Autodesk Inventor part; units mm, degrees
ref_plane "YZ Plane" through (0, 0, 0) normal (1, 0, 0) x (0, 1, 0)
ref_plane "XZ Plane" through (0, 0, 0) normal (0, 1, 0) x (-1, 0, 0)
ref_plane "XY Plane" through (0, 0, 0) normal (0, 0, 1) x (1, 0, 0)
sketch "Sketch1" plane through (0, 0, 0) normal (0, 0, 1) x (1, 0, 0)
  line L0 (-20, -5) -> (20, -5)
  line L1 (20, -5) -> (20, 5)
  line L2 (20, 5) -> (-20, 5)
  line L3 (-20, 5) -> (-20, -5)
  line L4 (-20, -5) -> (20, 5) construction
  line L5 (20, -5) -> (-20, 5) construction
  circle A0 centre (0, -18) radius 11.15
  circle A1 centre (0, -18) radius 5.25
  circle A2 centre (0, -18) radius 17.5
  line L6 (-20, -5) -> (-17.2455, -20.9738)
  line L7 (20, -5) -> (17.2455, -20.9738)
  circle A3 centre (0, -10) radius 1.65
  circle A4 centre (-8, -18) radius 1.65
  circle A5 centre (0, -26) radius 1.65
  circle A6 centre (8, -18) radius 1.65
  point P0 (0, 0)
  dimension "d0" = 22.3
  dimension "d1" = 10.5
  dimension "d2" = 35
  dimension "d3" = 3.3
  dimension "d4" = 8
  dimension "d7" = 360
  dimension "d14" = 40
  dimension "d16" = 23
  dimension "d17" = 10
extrude "Extrusion1" add sketch "Sketch1" along normal blind 10 contours L3 L2 L1 L0 A2 | L0 A2 L6 | A2 L0 | L0 A2 | L0 L7 A2 | A0
extrude "Extrusion2" cut sketch "Sketch1" along normal blind 3 contours A0
sketch "Sketch2" plane through (0, 0, 10) normal (0, 0, 1) x (1, 0, 0)
  line L0 (20, 5) -> (-20, 5)
  line L1 (-20, 5) -> (-20, -5)
  line L2 (-20, -5) -> (-17.2455, -20.9738)
  arc A0 (-17.2455, -20.9738) -> (17.2455, -20.9738) centre (0, -18) ccw
  line L3 (17.2455, -20.9738) -> (20, -5)
  line L4 (20, -5) -> (20, 5)
  circle A1 centre (0, -18) radius 5.25
  circle A2 centre (0, -10) radius 1.65
  circle A3 centre (-8, -18) radius 1.65
  circle A4 centre (0, -26) radius 1.65
  circle A5 centre (8, -18) radius 1.65
  circle A6 centre (-10, -3) radius 1.65
  circle A7 centre (10, -3) radius 1.65
  line L5 (-10, -3) -> (10, -3)
  point P0 (0, 0)
  point P1 (0, -3)
  dimension "d18" = 3.3
  dimension "d19" = 3.3
  dimension "d20" = 8
  dimension "d21" = 20
extrude "Extrusion3" cut sketch "Sketch2" against normal through all contours A6 | A7
properties part number "PARA_TUERCA" material "Steel, Mild, Welded"
Design review of the part built by this model. Coordinates are the model's own, in mm. A direction names the side the tool comes from. Give positions to 0.01 mm unless a question says otherwise; leave off trailing zeros. Loops run counter-clockwise (first coordinate to the right, second up) from the corner with the lowest first, then second, coordinate; pieces in that order, holes last. Notation, with made-up numbers: (70.25, -4) - (116.25, -4) arc R15 ccw to (116.25, 21) - close; hole circle Ø6 at (9, -3.75). An arc over 180 degrees is marked (long way). Write item = value, one per line.
1) Take a section at C-C on y = -13.5. State the section outline as (x, z) points.
Result sheet:
outline = (-18.53, 0) - (-10.2, 0) - (-10.2, 3) - (-2.7, 3) - (-2.7, 10) - (-18.53, 10) - close; (2.7, 3) - (10.2, 3) - (10.2, 0) - (18.53, 0) - (18.53, 10) - (2.7, 10) - close
2) Draft analysis for pull direction X (two halves, no side actions). For faces 1 (the face through (11.524, -3.632, 5.07)), 2 (the face through (20, 0, 5)), 3 (the face through (4, -10, 10)), state which applies: +X half, -X half, draft (parallel to the pull), parting line (faces both ways), or undercut.
Result sheet:
face_1 = undercut
face_2 = +X half
face_3 = draft
3) Clearance check with flat-ended pins moving along their axes: pin 1 Ø6 at (x, z) = (-14.5, 4) entering from -Y; pin 2 Ø1 at (y, z) = (-27.5, 3) entering from +X; pin 3 Ø6.5 at (x, y) = (-0.5, -15.5) entering from -Z. State where each tip first meets the part, or that it passes through.
Result sheet:
pin_1 = -31.19
pin_2 = 15.01
pin_3 = 3
4) Take a section at B-B on y = -3. State the section outline as (x, z) points, and give its area (3 significant figures).
Result sheet:
outline = (-20, 0) - (-11.65, 0) - (-11.65, 10) - (-20, 10) - close; (-8.35, 0) - (8.35, 0) - (8.35, 10) - (-8.35, 10) - close; (11.65, 0) - (20, 0) - (20, 10) - (11.65, 10) - close
area = 334 mm2
5) Take a section at D-D on x = -4.5. State the section outline as (y, z) points, and give its area (3 significant figures).
Result sheet:
outline = (-34.91, 0) - (-28.2, 0) - (-28.2, 3) - (-20.7, 3) - (-20.7, 10) - (-34.91, 10) - close; (-15.3, 3) - (-7.8, 3) - (-7.8, 0) - (5, 0) - (5, 10) - (-15.3, 10) - close
area = 300 mm2
6) Tool access review of faces 4 (the face through (-18.64, -12.88, 4.93)), 5 (the face through (6, -27.4, 1.5)): name each direction out of +Z, -Z, +X, -X, +Y, -Y from which nothing blocks a thin tool from reaching the whole face with its end or side.
Result sheet:
face_4 = +Z, -Z, -X, -Y
face_5 = -Z
7) Take a section at A-A on x = 0. State the section outline as (y, z) points.
Result sheet:
outline = (-35.5, 0) - (-29.15, 0) - (-29.15, 3) - (-27.65, 3) - (-27.65, 10) - (-35.5, 10) - close; (-24.35, 3) - (-23.25, 3) - (-23.25, 10) - (-24.35, 10) - close; (-12.75, 3) - (-11.65, 3) - (-11.65, 10) - (-12.75, 10) - close; (-8.35, 3) - (-6.85, 3) - (-6.85, 0) - (5, 0) - (5, 10) - (-8.35, 10) - close
8) To check wall thickness, follow line 1 (X direction, y = -2.5, z = 5.5); line 2 (Y direction, x = -9, z = 1.5); line 3 (Z direction, x = 6, y = -25). State the ranges of each line that lie inside material, in increasing order.
Result sheet:
line_1 = -20 to -11.57, -8.43 to 8.43, 11.57 to 20
line_2 = -33.01 to -24.58, -11.42 to -4.31, -1.69 to 5
line_3 = 3 to 10
